Read the model definition and answer for the solid it produces. Units are mm, in the model's axes. Face numbers are marked on the shaded views. Give positions to 0.01 mm unless a question says otherwise; leave off trailing zeros. Write each loop counter-clockwise with the first axis right and the second up, starting at its lowest first coordinate (ties: lowest second). Pieces come first, ordered by that corner, then holes. Notation, with made-up numbers: (12, -2.5) -> (71, -2.5) arc R25 cw to (71, 31.5) -> close; hole circle Ø8 at (27.5, 51.5). An arc over 180 degrees is marked (long way). Write item = value, one per line.
from build123d import *
from build123d.topology import SkipClean

# Parameters (mm, degrees)
BASPROSKE_W             = 8
BASPROSKE_H             = 12.25
TOOTHCUT_DEPTH          = 20.082059637
TEETHCUTS_COUNT         = 12
TEETHCUTS_ANGLE         = 330
HUBNEAONESKE_R          = 8.3115
HUBNEARONE_DEPTH        = 8.0000508
BORSKE_R                = 4.5
BORE_DEPTH              = 16.0000508
ESQUISSE1_R             = 8.3115
ENL_V_MAT_EXTRU_1_DEPTH = 8
ESQUISSE2_R             = 4.5
ESQUISSE2_R_2           = 4.275
BOSS_EXTRU_1_DEPTH      = 8
ESQUISSE3_R             = 4.6
ENL_V_MAT_EXTRU_2_DEPTH = 10


with BuildPart() as part:
    # BasProSke → Base-Revolve (revolve)
    with BuildSketch(Plane(origin=(0, 0, 0), x_dir=(1, 0, 0), z_dir=(0, 1, 0)), mode=Mode.PRIVATE) as base_revolve_sk:
        with Locations((4, 6.125)):
            Rectangle(BASPROSKE_W, BASPROSKE_H)
    revolve(base_revolve_sk.sketch.rotate(Axis((-10, 0, 0), (1, 0, 0)), 180), axis=Axis((-10, 0, 0), (1, 0, 0)))

    # TooCutSke → ToothCut (cut, through all)
    with BuildSketch(Plane(origin=(0, 0, 0), x_dir=(0, 0, -1), z_dir=(1, 0, 0))):
        with BuildLine():
            ThreePointArc((0.965128363, 8.255274647), (0, 8.3115), (-0.965128363, 8.255274647))
            ThreePointArc((-0.965128363, 8.255274647), (-1.43628674, 10.346733197), (-2.878284339, 11.933185846))
            ThreePointArc((-2.878284339, 11.933185846), (0, 12.2754), (2.878284339, 11.933185846))
            ThreePointArc((2.878284339, 11.933185846), (1.43628674, 10.346733197), (0.965128363, 8.255274647))
        make_face()
    toothcut = extrude(amount=TOOTHCUT_DEPTH, mode=Mode.SUBTRACT)

    # TeethCuts: ToothCut ×12 about axis
    teethcuts_axis = Axis((-10, 0, 0), (1, 0, 0))
    for i in range(1, TEETHCUTS_COUNT):
        add(toothcut.rotate(teethcuts_axis, i * TEETHCUTS_ANGLE / (TEETHCUTS_COUNT - 1)), mode=Mode.SUBTRACT)

    # HubNeaOneSke → HubNearOne (add)
    with SkipClean():  # the faces are left unmerged after this step: merging them gives an invalid solid
        with BuildSketch(Plane.ZY):
            Circle(HUBNEAONESKE_R)
        extrude(amount=HUBNEARONE_DEPTH)

    # BorSke → Bore (cut, symmetric)
    with SkipClean():  # the faces are left unmerged after this step: merging them gives an invalid solid
        with BuildSketch(Plane(origin=(0, 0, 0), x_dir=(0, 0, -1), z_dir=(1, 0, 0))):
            with Locations(Location((0, 0, 0), (0, 0, 180))):
                Circle(BORSKE_R)
        extrude(amount=BORE_DEPTH, both=True, mode=Mode.SUBTRACT)

    # Esquisse1 → Enlèv. mat.-Extru.1 (cut)
    with SkipClean():  # the faces are left unmerged after this step: merging them gives an invalid solid
        with BuildSketch(Plane.ZY.offset(8.0000508)):
            Circle(ESQUISSE1_R)
        extrude(amount=-ENL_V_MAT_EXTRU_1_DEPTH, mode=Mode.SUBTRACT)

    # Esquisse2 → Boss.-Extru.1 (add)
    with SkipClean():  # the faces are left unmerged after this step: merging them gives an invalid solid
        with BuildSketch(Plane(origin=(8, 0, 0), x_dir=(0, 0, -1), z_dir=(1, 0, 0))):
            with Locations(Location((0, 0, 0), (0, 0, 180))):
                Circle(ESQUISSE2_R)
            Circle(ESQUISSE2_R_2, mode=Mode.SUBTRACT)
        extrude(amount=-BOSS_EXTRU_1_DEPTH)

    # Esquisse3 → Enlèv. mat.-Extru.2 (cut)
    with SkipClean():  # the faces are left unmerged after this step: merging them gives an invalid solid
        with BuildSketch(Plane.ZY.offset(5.08e-05)):
            Circle(ESQUISSE3_R)
        extrude(amount=-ENL_V_MAT_EXTRU_2_DEPTH, mode=Mode.SUBTRACT)


solid = part.part
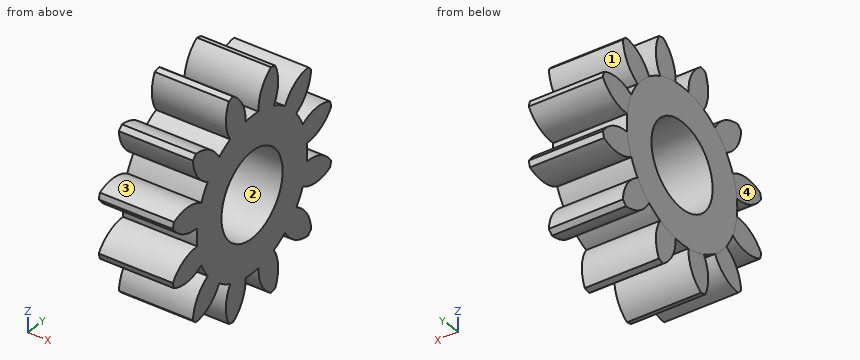
(1) Given P1, Ø2, axis at x = 5.5, z = 6, coming from the -Y side; P2, Ø12, axis at y = 0, z = 0, coming from the -X side; P3, Ø4, axis at x = 4, y = 9.5, coming from the -Z side; P4, Ø2, axis at x = 3, y = -5.5, coming from the +Z side, each flat-ended and moving along its own axis, determine where each tip first touches the part or whether it passes through.
Checks:
P1 = -8.55
P2 = 0
P3 = -8.89
P4 = 8.29
(2) Consider L1, parallel to Y at x = 5, z = -7; L2, parallel to Y at x = 4.5, z = -2.5; L3, parallel to Z at x = 7, y = 7.75. Determine where each line is inside the solid, lowest interval first.
Checks:
L1 = -8.55 to -5.16, -4.48 to 4.48, 5.16 to 8.55
L2 = -11.66 to -3.86, 3.86 to 11.66
L3 = -8.8 to -5.79, -3.36 to 3.36, 5.79 to 8.8
(3) For a pull along Y with two mould halves and no side action, classify the marked faces 1, 2, 3 and 4 as released by +Y, released by -Y, zero draft, split by the parting line, or undercut.
Checks:
face_1 = released by +Y
face_2 = undercut
face_3 = undercut
face_4 = zero draft
(4) The part is cut by section A-A on z = 0. Determine the outline of the cut face in (x, y), plus the area to 3 significant figures.
Checks:
outline = (0, -8.31) -> (8, -8.31) -> (8, -4.6) -> (0, -4.6) -> close; (0, 4.6) -> (8, 4.6) -> (8, 8.31) -> (0, 8.31) -> close
area = 59.4 mm²
